Can you work these out from the model? Positions are in its coordinate system, mm. Face numbers are marked on the shaded views. A direction names the side the tool comes from. Give positions to 0.01 mm unless a question says otherwise; leave off trailing zeros. Write each loop counter-clockwise with the first axis right and the second up, starting at its lowest first coordinate (ties: lowest second). Pieces come first, ordered by that corner, then holes.
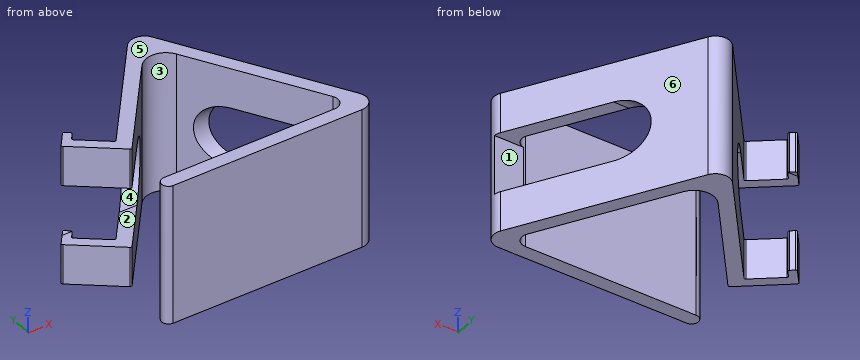
```python
from build123d import *

# Parameters (mm, degrees)
PAD_DEPTH         = 70
POCKET_DEPTH      = 75
POCKET_DEPTH_BACK = 65


with BuildPart() as part:
    # Sketch → Pad (new body)
    with BuildSketch(Plane.XY):
        with BuildLine():
            Line((-9.201384, 43.579781), (-46.391168, -2.578))
            ThreePointArc((-47.445741, -2.691469), (-46.894954, -2.853144), (-46.391168, -2.578))
            Line((-69.249206, 14.875799), (-47.445741, -2.691469))
            ThreePointArc((-69.362676, 15.930373), (-69.52435, 15.379586), (-69.249206, 14.875799))
            Line((-64.029755, 22.549282), (-69.362676, 15.930373))
            ThreePointArc((-62.975181, 22.662751), (-63.525968, 22.824426), (-64.029755, 22.549282))
            Line((-61.028444, 21.094245), (-62.975181, 22.662751))
            ThreePointArc((-60.914974, 20.039672), (-60.7533, 20.590459), (-61.028444, 21.094245))
            Line((-63.110883, 17.314239), (-60.914974, 20.039672))
            ThreePointArc((-63.110883, 17.314239), (-63.272557, 16.763452), (-62.997413, 16.259665))
            Line((-49.759595, 5.593824), (-62.997413, 16.259665))
            ThreePointArc((-49.759595, 5.593824), (-49.208808, 5.432149), (-48.705022, 5.707293))
            Line((-5.744258, 59.027676), (-48.705022, 5.707293))
            ThreePointArc((-5.744258, 59.027676), (0.368567, 61.665407), (5.998454, 58.111729))
            Line((53.504513, -24.375497), (5.998454, 58.111729))
            ThreePointArc((53.504513, -24.375497), (53.49727, -31.134135), (47.640508, -34.507202))
            Line((-47.756765, -34.405463), (47.640508, -34.507202))
            ThreePointArc((-47.631027, -27.500642), (-51.151742, -30.890084), (-47.756765, -34.405463))
            Line((-47.631027, -27.500642), (38.670947, -27.592682))
            ThreePointArc((38.670947, -27.592682), (43.12437, -25.027835), (43.129877, -19.888635))
            Line((43.129877, -19.888635), (7.319285, 42.291148))
            ThreePointArc((7.319285, 42.291148), (-0.60133, 47.290771), (-9.201384, 43.579781))
        make_face()
    extrude(amount=PAD_DEPTH)

    # Sketch001 → Pocket (cut, two sides)
    with BuildSketch(Plane.YZ) as pocket_sk:
        with BuildLine():
            Line((-27.500642, 50), (-27.500642, 20))
            Line((-27.500642, 20), (20.499358, 20))
            ThreePointArc((20.499358, 20), (35.499358, 35), (20.499358, 50))
            Line((20.499358, 50), (-27.500642, 50))
        make_face()
    extrude(amount=-POCKET_DEPTH, mode=Mode.SUBTRACT)
    extrude(pocket_sk.sketch, amount=POCKET_DEPTH_BACK, mode=Mode.SUBTRACT)


solid = part.part
```
1) Suppose I cut it at B-B on y = -22. Write out the boundary of the cut face in (x, z).
Values follow:
outline: (43.8, 0) - (52.14, 0) - (52.14, 20) - (43.8, 20) - close; (43.8, 50) - (52.14, 50) - (52.14, 70) - (43.8, 70) - close
2) If we mould it in two halves opening along Z, with no side actions, what happens to the marked faces 4, 5 and 6? For each: +Z half, -Z half, draft (parallel to the pull), parting line (faces both ways), or undercut.
Values follow:
face 4: undercut
face 5: +Z half
face 6: draft
3) Suppose I cut it at C-C on x = 25. Write out the boundary of the cut face in (y, z).
Values follow:
outline: (-34.48, 0) - (-27.58, 0) - (-27.58, 70) - (-34.48, 70) - close; (11.59, 0) - (25.12, 0) - (25.12, 20.73) arc R15 cw to (20.5, 20) - (11.59, 20) - close; (11.59, 50) - (20.5, 50) arc R15 cw to (25.12, 49.27) - (25.12, 70) - (11.59, 70) - close
4) Suppose I cut it at A-A on x = -11.5. Write out the boundary of the cut face in (y, z), plus the area to 3 significant figures.
Values follow:
outline: (-34.44, 0) - (-27.54, 0) - (-27.54, 70) - (-34.44, 70) - close; (40.73, 0) - (51.88, 0) - (51.88, 70) - (40.73, 70) - close
area: 1,260 mm2
5) For the marked faces 1, 2 and 3, which set-ups out of +Z, -Z, +X, -X, +Y, -Y let a thin tool reach every point of the face, with its end or its side?
Values follow:
face 1: +X, -X, +Y
face 2: +X, -X
face 3: +Z, -Z
6) Please list where these lines run through material, in increasing order: L1, parallel to Z at x = -32, y = 18; L2, parallel to X at y = 10, z = 15; L3, parallel to X at y = 32, z = 56.
Values follow:
L1: z = 0 to 20, 50 to 70
L2: x = -63.2 to -55.23, -45.25 to -36.26, 25.92 to 33.71
L3: x = -27.52 to -18.53, 13.25 to 21.04
7) For pin 1 Ø8 at (x, z) = (-43, 49) entering from +Y; pin 2 Ø8 at (x, y) = (-51.5, 7.5) entering from +Z; pin 3 Ø8 at (x, z) = (8.5, 54) entering from -Y; pin 4 Ø16 at (x, z) = (46.5, 30.5) entering from +Y, each with a flat end and sliding along its axis, tell me the tip position at first contact or that it passes through.
Values follow:
pin 1: stops at y = 17.59
pin 2: stops at z = 70
pin 3: stops at y = -34.47
pin 4: stops at y = -27.5
8) Suppose I cut it at D-D on z = 62.5. Write out the boundary of the cut face in (x, y).
Values follow:
outline: (-69.36, 15.93) arc R0.75 ccw to (-69.25, 14.88) - (-47.45, -2.69) arc R0.75 ccw to (-46.39, -2.58) - (-9.2, 43.58) arc R10.04 cw to (7.32, 42.29) - (43.13, -19.89) arc R5.14 cw to (38.67, -27.59) - (-47.63, -27.5) arc R3.45 ccw to (-47.76, -34.41) - (47.64, -34.51) arc R6.76 ccw to (53.5, -24.38) - (6, 58.11) arc R7.14 ccw to (-5.74, 59.03) - (-48.71, 5.71) arc R0.75 cw to (-49.76, 5.59) - (-63, 16.26) arc R0.75 cw to (-63.11, 17.31) - (-60.91, 20.04) arc R0.75 ccw to (-61.03, 21.09) - (-62.98, 22.66) arc R0.75 ccw to (-64.03, 22.55) - close
